from build123d import *

# Parameters (mm, degrees)
F0_W     = 65
F0_H     = 80
F1_DEPTH = 6
F2_R     = 5
F4_DEPTH = 3.1
F5_R     = 1.25
F6_DEPTH = 10
F8_D     = 15
F9_D     = 3.3


with BuildPart() as f1:
    # F0 (on Top) → F1 (new body)
    with BuildSketch(Plane.XY):
        Rectangle(F0_W, F0_H)
    extrude(amount=F1_DEPTH)

    # F2
    f2_edges = [f1.edges().sort_by_distance(p)[0] for p in [
        (32.5, -40, 3),
        (32.5, 40, 3),
        (-32.5, 40, 3),
        (-32.5, -40, 3),
    ]]
    fillet(f2_edges, radius=F2_R)

    # F3 (on face) → F4 (cut)
    with BuildSketch(Plane.XY.offset(6)):
        with BuildLine():
            Line((14, -40), (14, -5))
            ThreePointArc((14, -5), (0, 9), (-14, -5))
            Line((-14, -5), (-14, -40))
            Line((-14, -40), (14, -40))
        make_face()
    extrude(amount=-F4_DEPTH, mode=Mode.SUBTRACT)

    # F5 (on face) → F6 (join)
    with BuildSketch(Plane.XY.offset(2.9)):
        with Locations((0, -5)):
            Circle(F5_R)
        with Locations((0, -30)):
            Circle(F5_R)
    extrude(amount=F6_DEPTH)

    # F8 (through all)
    with Locations(Plane(origin=(0, 0, 0), x_dir=(1, 0, 0), z_dir=(0, 0, -1))):
        with Locations((0, -13)):
            Hole(F8_D / 2)

    # F9 (through all)
    with Locations(Plane(origin=(0, 0, 0), x_dir=(1, 0, 0), z_dir=(0, 0, -1))):
        with Locations((15.5, -28.5), (15.5, 2.5), (-15.5, 2.5), (-15.5, -28.5)):
            Hole(F9_D / 2)


solid = f1.part
Can you work these out from the model? Positions are in its coordinate system, mm. A direction names the side the tool comes from. Coordinates: 2 decimals unless noted, no trailing zeros. Order: outer loops, then holes, each group sorted by start corner. A loop starts at its lowest first (then second) coordinate and runs counter-clockwise, first axis right, second up. Notation, with made-up numbers: (46, -23) -> (80, -23) arc R14 cw to (80, 0) -> close; hole circle Ø4 at (3, 62). An arc over 180 degrees is marked (long way). Use one line per item in the form item = value.
Q1. Imagine slicing it at D-D, the plane z = 11.5. List the corners of the cut face in (x, y) for me, then the cut area to 3 significant figures.
From the geometry:
outline = circle Ø2.5 at (0, -30); circle Ø2.5 at (0, -5)
area = 9.82 mm²
Q2. I need wall thicknesses on L1, parallel to X at y = 28.5, z = 3.7; L2, parallel to Y at x = 15.5, z = 5.25; L3, parallel to X at y = -10, z = 5.5. Which ranges of each line are inside material? Lowest first, please.
From the geometry:
L1 = -32.5 to -17.15, -13.85 to 13.85, 17.15 to 32.5
L2 = -40 to -4.15, -0.85 to 26.85, 30.15 to 40
L3 = -32.5 to -14, 14 to 32.5
Q3. Will these pins go through, and if not, where does the flat tip stop? P1, Ø5, axis at x = -18.5, y = 13, coming from the +Z side; P2, Ø2, axis at x = -15.5, y = -2.5, coming from the +Z side.
From the geometry:
P1 = 6
P2 = through
Q4. Which directions (+Z, -Z, +X, -X, +Y, -Y) give clear straight access to the entire face, cutting with the end or side of a thin tool? Please do faces 4 (the face through (-0.27, -6.22, 7.83)), 5 (the face through (0, -5, 12.9)), 6 (the face through (-11.61, 2.82, 4.47)).
From the geometry:
face_4 = +Z
face_5 = +Z, +X, -X, +Y, -Y
face_6 = +Z, -Y
Q5. Imagine slicing it at A-A, the plane y = 13. List the corners of the cut face in (x, z) for me, then the cut area to 3 significant figures.
From the geometry:
outline = (-32.5, 0) -> (-7.5, 0) -> (-7.5, 6) -> (-32.5, 6) -> close; (7.5, 0) -> (32.5, 0) -> (32.5, 6) -> (7.5, 6) -> close
area = 300 mm²
Q6. Imagine slicing it at B-B, the plane z = 2. List the corners of the cut face in (x, y) for me.
From the geometry:
outline = (-32.5, -35) arc R5 ccw to (-27.5, -40) -> (27.5, -40) arc R5 ccw to (32.5, -35) -> (32.5, 35) arc R5 ccw to (27.5, 40) -> (-27.5, 40) arc R5 ccw to (-32.5, 35) -> close; hole circle Ø3.3 at (-15.5, -2.5); hole circle Ø3.3 at (-15.5, 28.5); hole circle Ø15 at (0, 13); hole circle Ø3.3 at (15.5, -2.5); hole circle Ø3.3 at (15.5, 28.5)
Q7. We'd pull the mould along Y, two halves only. Please class faces 1 (the face through (-8, 9, 6)), 2 (the face through (0, -40, 2)), 3 (the face through (-16.39, 27.11, 3.04)): released by +Y, released by -Y, zero draft, split by the parting line, or undercut.
From the geometry:
face_1 = zero draft
face_2 = released by -Y
face_3 = undercut
Q8. Imagine slicing it at C-C, the plane x = 0. List the corners of the cut face in (y, z) for me.
From the geometry:
outline = (-40, 0) -> (5.5, 0) -> (5.5, 2.9) -> (-3.75, 2.9) -> (-3.75, 12.9) -> (-6.25, 12.9) -> (-6.25, 2.9) -> (-28.75, 2.9) -> (-28.75, 12.9) -> (-31.25, 12.9) -> (-31.25, 2.9) -> (-40, 2.9) -> close; (20.5, 0) -> (40, 0) -> (40, 6) -> (20.5, 6) -> close
